Read the model definition and answer for the solid it produces. Units are mm, in the model's axes. Face numbers are marked on the shaded views. A direction names the side the tool comes from. Give positions to 0.01 mm unless a question says otherwise; leave off trailing zeros. Write each loop counter-clockwise with the first axis right and the second up, starting at its lowest first coordinate (ties: lowest second). Pieces come first, ordered by that corner, then holes. Notation, with made-up numbers: M 81,25 L 131,25 A21 ccw 131,45 Z; hole C 47,-19.5 d9. An arc over 180 degrees is marked long. Put each result on its own line as item: value.
from build123d import *

# Parameters (mm, degrees)
SKETCH1_R                   = 60
BOSS_EXTRUDE1_DEPTH         = 7
SKETCH2_R                   = 10.25
CUT_EXTRUDE1_DEPTH          = 1.5
TAP_DRILL_FOR_M2X0_4_TAP1_D = 1.6
CIRPATTERN1_COUNT           = 4
SKETCH8_R                   = 35
SKETCH8_R_2                 = 25
CUT_EXTRUDE_THIN1_DEPTH     = 4


with BuildPart() as part:
    # Sketch1 → Boss-Extrude1 (new body)
    with BuildSketch(Plane(origin=(0, 0, 0), x_dir=(1, 0, 0), z_dir=(0, 1, 0))):
        with Locations(Location((0, 0, 0), (0, 0, 270))):
            Circle(SKETCH1_R)
    extrude(amount=BOSS_EXTRUDE1_DEPTH)

    # Sketch2 → Cut-Extrude1 (cut)
    with BuildSketch(Plane(origin=(0, 7, 0), x_dir=(1, 0, 0), z_dir=(0, 1, 0))):
        with Locations(Location((0, 0, 0), (0, 0, 270))):
            Circle(SKETCH2_R)
    extrude(amount=-CUT_EXTRUDE1_DEPTH, mode=Mode.SUBTRACT)

    # Tap Drill for M2x0.4 Tap1 (through all)
    with Locations(Plane(origin=(0, 5.5, 0), x_dir=(1, 0, 0), z_dir=(0, 1, 0))):
        with Locations((0, 8)):
            tap_drill_for_m2x0_4_tap1 = Hole(TAP_DRILL_FOR_M2X0_4_TAP1_D / 2)

    # CirPattern1: Tap Drill for M2x0.4 Tap1 ×4 about axis
    cirpattern1_axis = Axis((0, 0, 0.049031578), (0, 1, 0))
    for i in range(1, CIRPATTERN1_COUNT):
        add(tap_drill_for_m2x0_4_tap1.rotate(cirpattern1_axis, i * 360 / CIRPATTERN1_COUNT), mode=Mode.SUBTRACT)

    # Sketch8 → Cut-Extrude-Thin1 (cut)
    with BuildSketch(Plane.XZ):
        Circle(SKETCH8_R)
        Circle(SKETCH8_R_2, mode=Mode.SUBTRACT)
    extrude(amount=-CUT_EXTRUDE_THIN1_DEPTH, mode=Mode.SUBTRACT)


solid = part.part
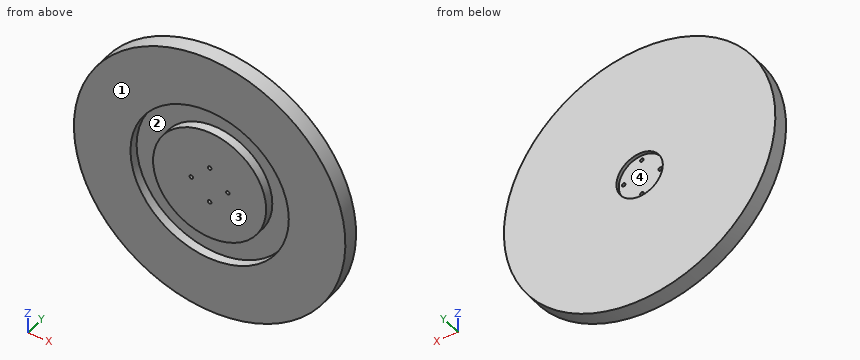
(1) Given pin 1 Ø1.3 at (x, z) = (0, -8) entering from -Y; pin 2 Ø1 at (x, y) = (-19.5, 1.5) entering from -Z; pin 3 Ø2 at (x, z) = (8.05, 0.05) entering from +Y; pin 4 Ø1.5 at (x, y) = (-44, 1) entering from -Z, each flat-ended and moving along its own axis, determine where each tip first touches the part or whether it passes through.
Result:
pin 1: passes through
pin 2: stops at z = -56.91
pin 3: stops at y = 5.5
pin 4: stops at z = -41.59
(2) Section C-C on x = 23.5 is taken. Determine the outline of the cut face in (y, z), and give its area (3 significant figures).
Result:
outline: M 0,-55.21 L 7,-55.21 L 7,55.21 L 0,55.21 L 0,25.94 L 4,25.94 L 4,8.53 L 0,8.53 L 0,-8.53 L 4,-8.53 L 4,-25.94 L 0,-25.94 Z
area: 634 mm²
(3) Section A-A on y = 2.25 is taken. Determine the outline of the cut face in (x, z).
Result:
outline: C 0,0 d120; C 0,0 d50; hole C 0,0 d70; hole C -8.05,0.05 d1.6; hole C 0,-8 d1.6; hole C 0,8.1 d1.6; hole C 8.05,0.05 d1.6
(4) Straight lines are drawn through the part: line 1 along Z through (x, y) = (2.5, 2.5); line 2 along Z through (x, y) = (5.5, 2.5); line 3 along X through (y, z) = (2.5, -4.5). For each, find the intervals that lie inside material, in ascending order. Write a range as from..to.
Result:
line 1: z = -59.95..-34.91, -24.87..24.87, 34.91..59.95
line 2: z = -59.75..-34.57, -24.39..24.39, 34.57..59.75
line 3: x = -59.83..-34.71, -24.59..24.59, 34.71..59.83
(5) Which of the six approach directions +Z, -Z, +X, -X, +Y, -Y give full straight-line access (tool end or side, diameter ignored) to the marked faces 1 and 2?
Result:
face 1: +Z, -Z, +X, -X, -Y
face 2: -Y
(6) Section B-B on z = -17 is taken. Determine the outline of the cut face in (x, y).
Result:
outline: M -57.54,0 L -30.59,0 L -30.59,4 L -18.33,4 L -18.33,0 L 18.33,0 L 18.33,4 L 30.59,4 L 30.59,0 L 57.54,0 L 57.54,7 L -57.54,7 Z
(7) Section D-D on z = -31.5 is taken. Determine the outline of the cut face in (x, y).
Result:
outline: M -51.07,0 L -15.26,0 L -15.26,4 L 15.26,4 L 15.26,0 L 51.07,0 L 51.07,7 L -51.07,7 Z
(8) For a pull along Z with two mould halves and no side action, classify the marked faces 3 and 4 as +Z half, -Z half, draft (parallel to the pull), parting line (faces both ways), or undercut.
Result:
face 3: draft
face 4: undercut
